Geometry check sheet. Reference: drawing and pictorial views, mm from the part's lowest x, y, z. A direction names the side the tool comes from. Round coordinates to 2 decimals unless told otherwise and drop trailing zeros. Write each loop counter-clockwise with the first axis right and the second up, starting at its lowest first coordinate (ties: lowest second). Pieces come first, ordered by that corner, then holes. Notation, with made-up numbers: (22.25, 40) - (30.25, 40) arc R22 cw to (30.25, 52) - close; hole circle Ø11 at (69, -9). An arc over 180 degrees is marked (long way). Return JSON: item names as keys, results as strings.
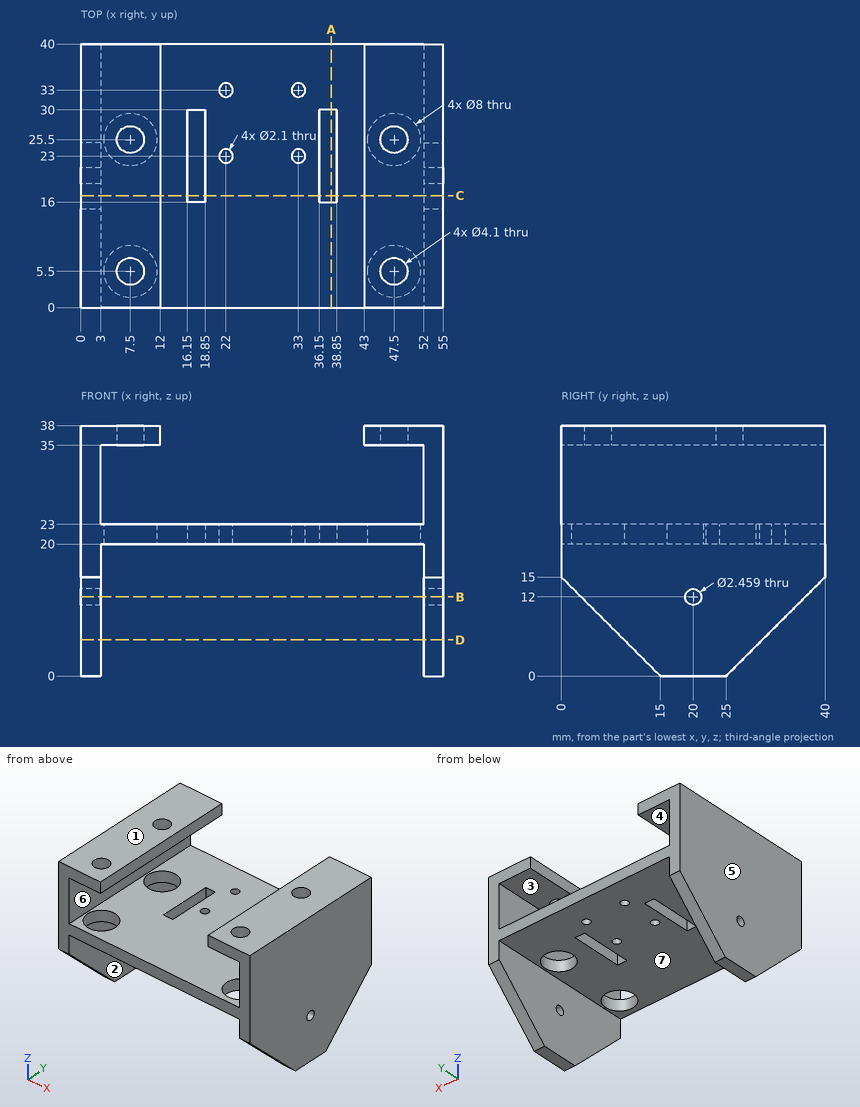
(1) Section check D-D, the plane z = 5.5. Enter the section's corners in (x, y), plus the area to 3 significant figures.
Response values:
{"outline": "(0, 9.5) - (3, 9.5) - (3, 30.5) - (0, 30.5) - close; (52, 9.5) - (55, 9.5) - (55, 30.5) - (52, 30.5) - close", "area": "126 mm^2"}
(2) Section check C-C, the plane y = 17. Enter the section's corners in (x, z), plus the area to 3 significant figures.
Response values:
{"outline": "(0, 0) - (3, 0) - (3, 20) - (16.15, 20) - (16.15, 23) - (3, 23) - (3, 35) - (12, 35) - (12, 38) - (0, 38) - close; (18.85, 20) - (36.15, 20) - (36.15, 23) - (18.85, 23) - close; (38.85, 20) - (52, 20) - (52, 0) - (55, 0) - (55, 38) - (43, 38) - (43, 35) - (52, 35) - (52, 23) - (38.85, 23) - close", "area": "413 mm^2"}
(3) Section check A-A, the plane x = 38. Enter the section's corners in (y, z).
Response values:
{"outline": "(0, 20) - (16, 20) - (16, 23) - (0, 23) - close; (30, 20) - (40, 20) - (40, 23) - (30, 23) - close"}
(4) Access from +Z, -Z, +X, -X, +Y, -Y to the whole of each face (thin tool, end or side, straight path). Record for the marked faces 5, 6 and 7.
Response values:
{"face 5": "+Z, -Z, -X, +Y, -Y", "face 6": "+Y, -Y", "face 7": "-Z, +Y, -Y"}
(5) Release check for a two-part mould opening along Z. For the marked faces 1, 2, 3 and 4 record: pulls with the +Z half, pulls with the -Z half, needs draft (parallel to the pull), parting line crosses it, or undercut.
Response values:
{"face 1": "pulls with the +Z half", "face 2": "needs draft", "face 3": "undercut", "face 4": "undercut"}
(6) Gauge pin test, flat ends, axial feed: pin 1 (2 mm diameter, centred on y = 20, z = 12, fed in from +X); pin 2 (2 mm diameter, centred on x = 31.5, y = 19.5, fed in from +Z); pin 3 (10 mm diameter, centred on x = 49, y = 10.5, fed in from -Z); pin 4 (12 mm diameter, centred on x = 34.5, y = 28.5, fed in from -Z). Record the tip position at first contact, or that the pin passes through.
Response values:
{"pin 1": "passes through", "pin 2": "stops at z = 23", "pin 3": "stops at z = 0.5", "pin 4": "stops at z = 20"}
(7) Material ranges on line 1 along X through (y, z) = (33, 20.75); line 2 along X through (y, z) = (5.5, 36); line 3 along Y through (x, z) = (47.5, 36.8), recorded low to high. Write a range as [from, to].
Response values:
{"line 1": "x = [0, 20.95], [23.05, 31.95], [34.05, 55]", "line 2": "x = [0, 5.45], [9.55, 12], [43, 45.45], [49.55, 55]", "line 3": "y = [0, 3.45], [7.55, 23.45], [27.55, 40]"}
(8) Section check B-B, the plane z = 12. Enter the section's corners in (x, y), plus the area to 3 significant figures.
Response values:
{"outline": "(0, 3) - (3, 3) - (3, 18.77) - (0, 18.77) - close; (0, 21.23) - (3, 21.23) - (3, 37) - (0, 37) - close; (52, 3) - (55, 3) - (55, 18.77) - (52, 18.77) - close; (52, 21.23) - (55, 21.23) - (55, 37) - (52, 37) - close", "area": "189 mm^2"}
